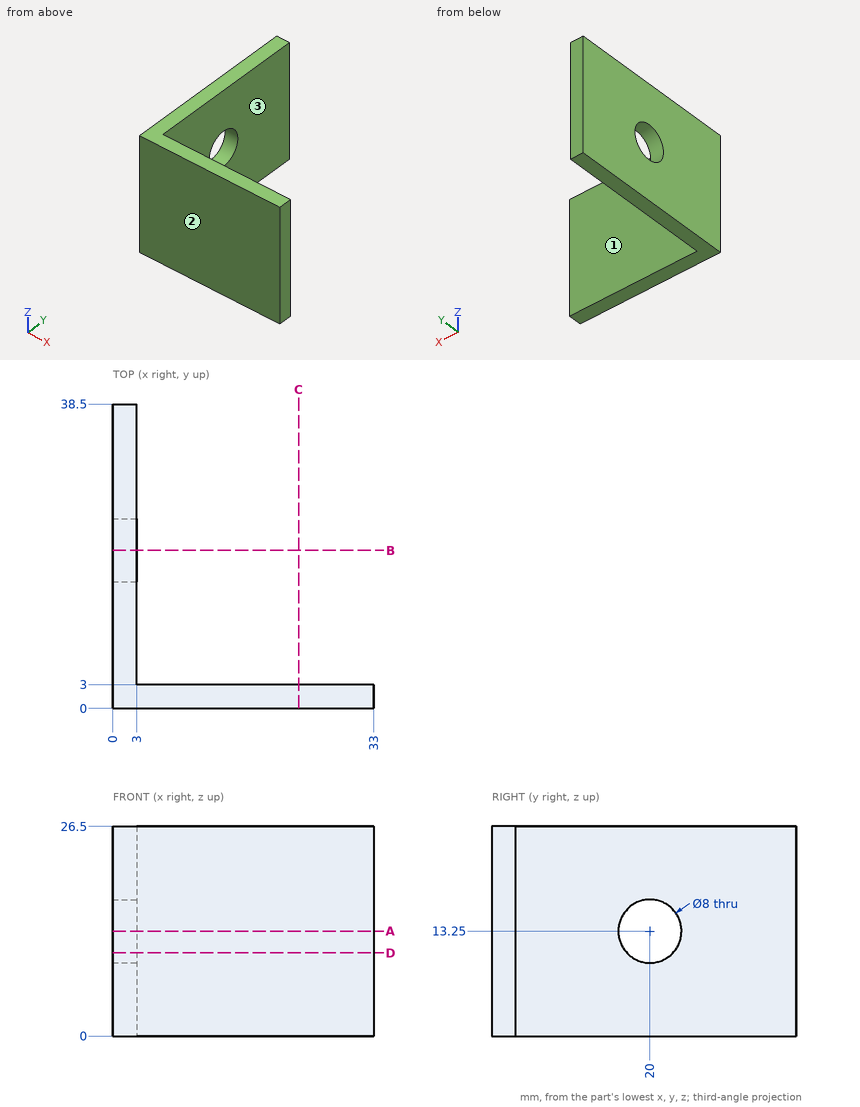
Design review of the part shown in the three views and the two pictorial views. Dimensions are in mm from the part's minimum x, y and z. Round coordinates to 2 decimals unless told otherwise and drop trailing zeros. Order: outer loops, then holes, each group sorted by start corner. A loop starts at its lowest first (then second) coordinate and runs counter-clockwise, first axis right, second up. Notation, with made-up numbers: (-34, 19) -> (12, 19) arc R29 cw to (12, 52) -> close; hole circle Ø4 at (-35.5, 8.5). An arc over 180 degrees is marked (long way). Write item = value, one per line. Start each with the question number.
1) To check wall thickness, follow line 1 (Z direction, x = 2.15, y = 20); line 2 (Y direction, x = 1.1, z = 13.25); line 3 (Y direction, x = 8.5, z = 22.5). State the ranges of each line that lie inside material, in increasing order. Write a range as from..to.
2) Insertion check: pin 1 (1.5 mm diameter, centred on x = 3.5, z = 10, fed in from -Y); pin 2 (13 mm diameter, centred on y = 20, z = 13.25, fed in from +X); pin 3 (13 mm diameter, centred on x = 20.5, z = 17, fed in from +Y); pin 4 (5 mm diameter, centred on x = 7, y = 25.5, fed in from -Z). Each pin has a flat end and moves straight along its axis. Give the tip position at first contact, or say it passes through.
3) Take a section at C-C on x = 23.5. State the section outline as (y, z) points.
4) The part is to be moulded in two halves that separate along Y. For the marked faces 1, 2 and 3, say which applies: +Y half, -Y half, draft (parallel to the pull), parting line (faces both ways), or undercut.
5) Take a section at B-B on y = 20. State the section outline as (x, z) points, plus the area to 3 significant figures.
6) Take a section at D-D on z = 10.5. State the section outline as (x, y) points, plus the area to 3 significant figures.
7) Take a section at A-A on z = 13.25. State the section outline as (x, y) points.
Verdict:
q1.line_1 = 0..9.25, 17.25..26.5
q1.line_2 = 0..16, 24..38.5
q1.line_3 = 0..3
q2.pin_1 = 0
q2.pin_2 = 3
q2.pin_3 = 3
q2.pin_4 = through
q3.outline = (0, 0) -> (3, 0) -> (3, 26.5) -> (0, 26.5) -> close
q4.face_1 = +Y half
q4.face_2 = -Y half
q4.face_3 = draft
q5.outline = (0, 0) -> (3, 0) -> (3, 9.25) -> (0, 9.25) -> close; (0, 17.25) -> (3, 17.25) -> (3, 26.5) -> (0, 26.5) -> close
q5.area = 55.5 mm2
q6.outline = (0, 0) -> (33, 0) -> (33, 3) -> (3, 3) -> (3, 17.1) -> (0, 17.1) -> close; (0, 22.9) -> (3, 22.9) -> (3, 38.5) -> (0, 38.5) -> close
q6.area = 188 mm2
q7.outline = (0, 0) -> (33, 0) -> (33, 3) -> (3, 3) -> (3, 16) -> (0, 16) -> close; (0, 24) -> (3, 24) -> (3, 38.5) -> (0, 38.5) -> close
